Build history of the part. All positions in model axes, mm. Face numbers are marked on the shaded views. A direction names the side the tool comes from. Round coordinates to 2 decimals unless told otherwise and drop trailing zeros. Loops run counter-clockwise (first coordinate to the right, second up) from the corner with the lowest first, then second, coordinate; pieces in that order, holes last. Notation, with made-up numbers: (5, 75) - (39, 75) arc R14 cw to (39, 94) - close; hole circle Ø2 at (3.25, 71). An arc over 180 degrees is marked (long way). One line per question, with ' | ' between items. Start each with the question number.
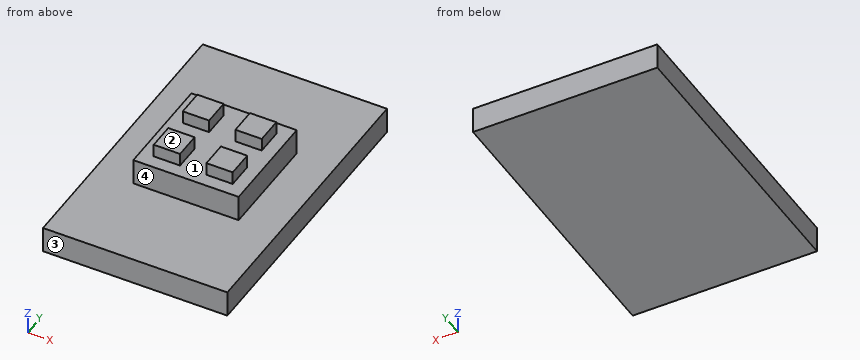
from build123d import *

# Parameters (mm, degrees)
F0_W     = 70
F0_H     = 110
F1_DEPTH = 10
F2_W     = 40
F2_H     = 40
F3_DEPTH = 10
F4_W     = 10
F4_H     = 10
F5_DEPTH = 5


with BuildPart() as f1:
    # F0 (on Top) → F1 (new body)
    with BuildSketch(Plane.XY):
        Rectangle(F0_W, F0_H)
    extrude(amount=F1_DEPTH)

    # F2 (on face) → F3 (join)
    with BuildSketch(Plane.XY.offset(10)):
        Rectangle(F2_W, F2_H)
    extrude(amount=F3_DEPTH)

    # F4 (on face) → F5 (join)
    with BuildSketch(Plane.XY.offset(20)):
        with Locations((-10, 10)):
            Rectangle(F4_W, F4_H)
        with Locations((10, 10)):
            Rectangle(F4_W, F4_H)
        with Locations((10, -10)):
            Rectangle(F4_W, F4_H)
        with Locations((-10, -10)):
            Rectangle(F4_W, F4_H)
    extrude(amount=F5_DEPTH)


solid = f1.part
1) Saw through at B-B on y = 36. Write the cut outline in (x, z).
2) Two-plate mould, pull along X, no slides. Class the marked faces 1 and 2: +X half, -X half, draft (parallel to the pull), parting line (faces both ways), or undercut.
3) Wall check: line 1 (Z direction, x = -23.5, y = -12.5); line 2 (Y direction, x = -8.5, z = 24.25); line 3 (Y direction, x = -11.5, z = 15.25). Give the ranges that are in metal, low to high. Write a range as [from, to].
4) Saw through at C-C on x = -10. Write the cut outline in (y, z).
5) Saw through at A-A on x = -1.5. Write the cut outline in (y, z).
6) Saw through at D-D on z = 14. Write the cut outline in (x, y).
7) Tool access for the marked faces 3 and 4: list every direction of +Z, -Z, +X, -X, +Y, -Y with a clear straight run to the whole face (end or side of a thin tool).
8) Drop flat-ended pins along their axis: pin 1 (1.5 mm diameter, centred on y = -12, z = 22, fed in from +X); pin 2 (2.5 mm diameter, centred on x = -12.5, z = 23, fed in from +Y); pin 3 (1.5 mm diameter, centred on x = 7.5, z = 22.5, fed in from -Y). Give the stop position or say it passes through.
Answer key:
1) outline: (-35, 0) - (35, 0) - (35, 10) - (-35, 10) - close
2) face 1: undercut | face 2: draft
3) line 1: [0, 10] | line 2: [-15, -5], [5, 15] | line 3: [-20, 20]
4) outline: (-55, 0) - (55, 0) - (55, 10) - (20, 10) - (20, 20) - (15, 20) - (15, 25) - (5, 25) - (5, 20) - (-5, 20) - (-5, 25) - (-15, 25) - (-15, 20) - (-20, 20) - (-20, 10) - (-55, 10) - close
5) outline: (-55, 0) - (55, 0) - (55, 10) - (20, 10) - (20, 20) - (-20, 20) - (-20, 10) - (-55, 10) - close
6) outline: (-20, -20) - (20, -20) - (20, 20) - (-20, 20) - close
7) face 3: +Z, -Z, +X, -X, -Y | face 4: +Z, +X, -X, -Y
8) pin 1: x = 15 | pin 2: y = 15 | pin 3: y = -15
